Read the model definition and answer for the solid it produces. Units are mm, in the model's axes. A direction names the side the tool comes from. Coordinates: 2 decimals unless noted, no trailing zeros. Order: outer loops, then holes, each group sorted by start corner. A loop starts at its lowest first (then second) coordinate and runs counter-clockwise, first axis right, second up. Notation, with made-up numbers: M -34.5,-34 L 13.5,-34 A17 cw 13.5,-25 Z; hole C 14.25,78.25 d11. An arc over 180 degrees is marked long. Use a Markdown table: item, result. Add a question column.
1) Find section D-D on z = -5. Write down the section's boundary in (x, y), plus the area to 3 significant figures.
2) Find section A-A on y = 15. Write down the section's boundary in (x, z).
3) Find section C-C on y = 2.25. Write down the section's boundary in (x, z).
4) Find section B-B on x = 4.5. Write down the section's boundary in (y, z).
5) Find the intervals of material crossed by probe 1 along Y at (x, z) = (4.5, -17); probe 2 along X at (y, z) = (7, -5); probe 3 along X at (y, z) = (8.25, -31.5), in increasing order. Write a range as [from, to].
6) This flat-tipped pin is pushed along its axis until it touches: pin 1 Ø2 at (x, z) = (18, -24.5) entering from -Y. Where does it stop, or does it pass through?
7) For faces 1 (the face through (0, 10, -17)), 2 (the face through (13, 10, -5)), determine the directions among +Z, -Z, +X, -X, +Y, -Y from which every point of the face is accessible in a straight line to the end or side of a thin tool.
8) The mould has two halves that part along Z. Classify faces 3 (the face through (14.397, 4.93, -31.21)), 4 (the face through (5.68, 12.74, -17.26)), 5 (the face through (12, 10, -35)): released by +Z, released by -Z, zero draft, split by the parting line, or undercut.
from build123d import *

# Parameters (mm, degrees)
SKETCH1_W           = 25
SKETCH1_H           = 35
BOSS_EXTRUDE1_DEPTH = 20
SKETCH3_R           = 2.55
CUT_EXTRUDE2_DEPTH  = 48.434164903
SKETCH4_R           = 2.25
CUT_EXTRUDE3_DEPTH  = 10


with BuildPart() as part:
    # Sketch1 → Boss-Extrude1 (new body)
    with BuildSketch(Plane(origin=(0, 0, 0), x_dir=(1, 0, 0), z_dir=(0, 1, 0))):
        with Locations((12.5, 17.5)):
            Rectangle(SKETCH1_W, SKETCH1_H)
    extrude(amount=BOSS_EXTRUDE1_DEPTH)

    # Sketch3 → Cut-Extrude2 (cut, through all)
    with BuildSketch(Plane.XY):
        with Locations((4.5, 15)):
            Circle(SKETCH3_R)
        with Locations((20.5, 15)):
            Circle(SKETCH3_R)
    extrude(amount=-CUT_EXTRUDE2_DEPTH, mode=Mode.SUBTRACT)

    # Sketch4 → Cut-Extrude3 (cut)
    with BuildSketch(Plane.XZ):
        with Locations(Location((12.5, -5, 0), (0, 0, 270))):
            Circle(SKETCH4_R)
        with Locations(Location((12.5, -30, 0), (0, 0, 270))):
            Circle(SKETCH4_R)
    extrude(amount=-CUT_EXTRUDE3_DEPTH, mode=Mode.SUBTRACT)


solid = part.part
Check result:
| question | item | result |
|---|---|---|
| 1 | outline | M 0,0 L 10.25,0 L 10.25,10 L 14.75,10 L 14.75,0 L 25,0 L 25,20 L 0,20 Z; hole C 4.5,15 d5.1; hole C 20.5,15 d5.1 |
| 1 | area | 414 mm2 |
| 2 | outline | M 0,-35 L 1.95,-35 L 1.95,0 L 0,0 Z; M 7.05,-35 L 17.95,-35 L 17.95,0 L 7.05,0 Z; M 23.05,-35 L 25,-35 L 25,0 L 23.05,0 Z |
| 3 | outline | M 0,-35 L 25,-35 L 25,0 L 0,0 Z; hole C 12.5,-30 d4.5; hole C 12.5,-5 d4.5 |
| 4 | outline | M 0,-35 L 12.45,-35 L 12.45,0 L 0,0 Z; M 17.55,-35 L 20,-35 L 20,0 L 17.55,0 Z |
| 5 | probe 1 | y = [0, 12.45], [17.55, 20] |
| 5 | probe 2 | x = [0, 10.25], [14.75, 25] |
| 5 | probe 3 | x = [0, 10.82], [14.18, 25] |
| 6 | pin 1 | stops at y = 0 |
| 7 | face 1 | +Z, -Z, -X, +Y, -Y |
| 7 | face 2 | -Y |
| 8 | face 3 | undercut |
| 8 | face 4 | zero draft |
| 8 | face 5 | released by -Z |
